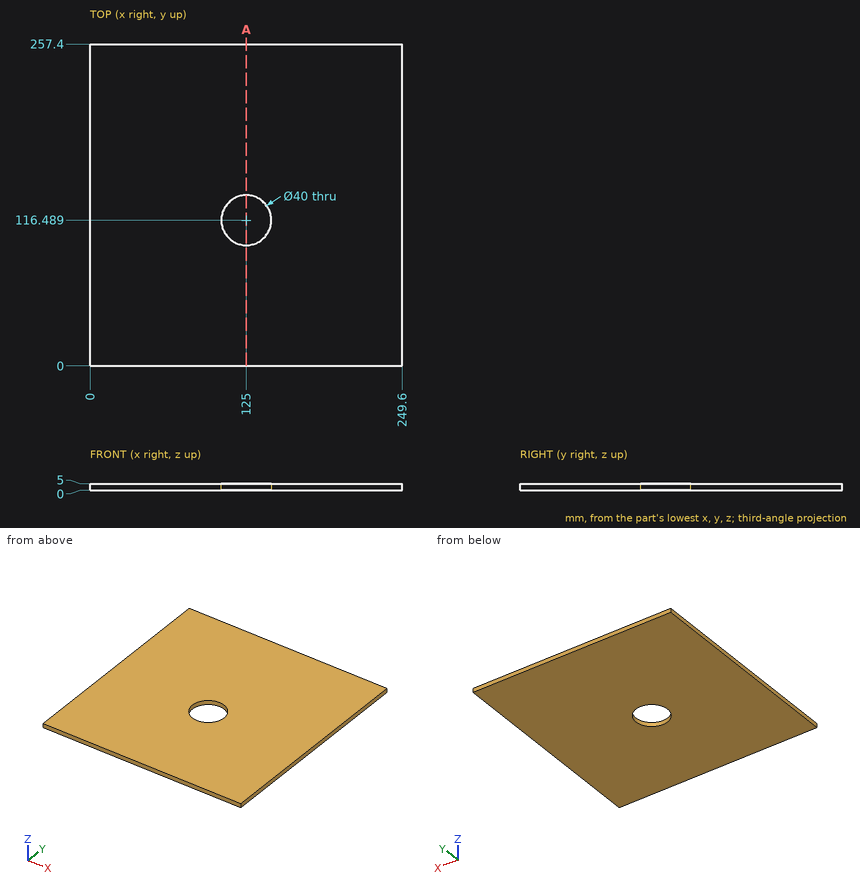
Design review of the part shown in the three views and the two pictorial views. Dimensions are in mm from the part's minimum x, y and z. Give positions to 0.01 mm unless a question says otherwise; leave off trailing zeros. Loops run counter-clockwise (first coordinate to the right, second up) from the corner with the lowest first, then second, coordinate; pieces in that order, holes last. Notation, with made-up numbers: (89.25, -32.5) -> (99.25, -32.5) arc R20 ccw to (99.25, -11.5) -> close; hole circle Ø3 at (62.25, -38). An arc over 180 degrees is marked (long way). Answer as a JSON object with one key per item and string values. Group by question number.
Q1. Wall thickness on line 1 along Y through (x, z) = (125, 3.9); line 2 along X through (y, z) = (117, 3.35); line 3 along Y through (x, z) = (120, 4.2): over which ranges is each line inside the solid? List them lowest first.
Q2. Take a section at A-A (x = 125). Write out the cut boundary in (y, z).
Q3. Insertion check: pin 1 (3 mm diameter, centred on x = 35.5, y = 175.5, fed in from -Z). The pin has a flat end and moves straight along its axis. Give the tip position at first contact, or say it passes through.
Answer below:
{
 "1": {"line 1": "y = 0 to 96.49, 136.49 to 257.4", "line 2": "x = 0 to 105.01, 144.99 to 249.6", "line 3": "y = 0 to 97.12, 135.85 to 257.4"},
 "2": {"outline": "(0, 0) -> (96.49, 0) -> (96.49, 5) -> (0, 5) -> close; (136.49, 0) -> (257.4, 0) -> (257.4, 5) -> (136.49, 5) -> close"},
 "3": {"pin 1": "stops at z = 0"}
}
